```python
from build123d import *

# Parameters (mm, degrees)
F1_DEPTH = 60


# Not quite as in the source:
# - a feature names something its author has since deleted; it is built from what else it names


with BuildPart() as f1:
    # F0 (on Right) → F1 (new body)
    with BuildSketch(Plane.YZ):
        Polygon((-9.6511039816, 84.8569979519), (11.5631884334, -16.6570162717), (-54.0677122772, -34.3161821365), (58.7390847504, -34.3161821365), (57.1931600571, -30.1430020481), (52.030442059, -16.6570162717), (41.619012037, -7.4873352069), (45.6172674894, -16.6570162717), (45.6120451947, -16.6570162717), (34.6120451947, -16.6570162717), align=None)
        Polygon((-33.4832413232, -32.6066525748), (14.5474322128, -19.683142134), (1.6078982385, -32.6066525748), align=None, mode=Mode.SUBTRACT)
        Polygon((6.7093357808, -32.6066525748), (27.5331988357, -11.8085765279), (36.6017826139, -32.6066525748), align=None, mode=Mode.SUBTRACT)
        Polygon((34.5994135062, -18.9948312665), (45.6120451947, -18.9948312665), (49.0652749053, -18.9948312665), (54.2761653822, -32.6066525748), (40.534575087, -32.6066525748), (38.136206347, -27.1061845124), align=None, mode=Mode.SUBTRACT)
        Polygon((16.4317106992, -17.8011970237), (3.8088566841, 42.6013163841), (25.9855565835, -8.2591820422), align=None, mode=Mode.SUBTRACT)
    extrude(amount=F1_DEPTH)


solid = f1.part
```
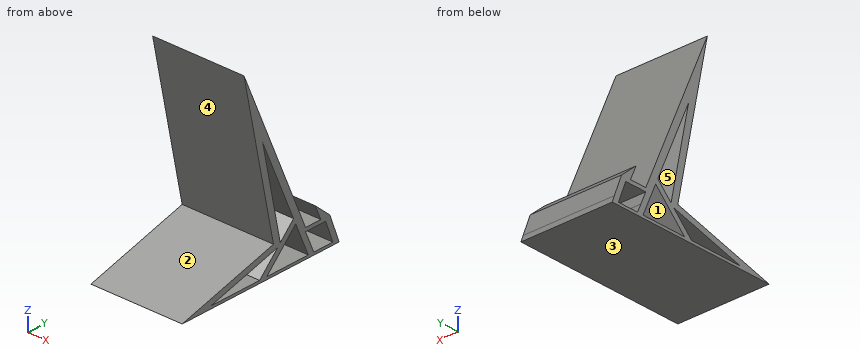
Geometry: final body of the model. Coordinates: model frame, mm. Face numbers are marked on the shaded views. A direction names the side the tool comes from. Round coordinates to 2 decimals unless told otherwise and drop trailing zeros. Order: outer loops, then holes, each group sorted by start corner. A loop starts at its lowest first (then second) coordinate and runs counter-clockwise, first axis right, second up. Notation, with made-up numbers: (-7, -13) -> (27, -13) arc R3 cw to (27, -9) -> close; hole circle Ø3 at (-18.75, 29.5). An arc over 180 degrees is marked (long way). Use one line per item in the form item = value. Start each with the question number.
1. Pin query (flat end, axial travel): pin 1 Ø4 at (x, y) = (47, -12) entering from +Z; pin 2 Ø6 at (x, z) = (8, 26) entering from -Y; pin 3 Ø4 at (x, y) = (44.5, 16.5) entering from +Z. Return the tip coordinate at first contact, or that it passes through.
2. Cut plane C-C (y = -6.5). Return the cut outline in (x, z), then the cut area to 3 significant figures.
3. Cut plane B-B (y = 13). Return the cut outline in (x, z), then the cut area to 3 significant figures.
4. Line query: probe 1 along Y at (x, z) = (45, -13); probe 2 along Z at (x, y) = (45, 25.5); probe 3 along Z at (x, y) = (20.5, -17). Output: solid intervals per line, ascending.
5. Draft query along Y for the marked faces 3, 4 and 5. Return one class per face: pulls with the +Y half, pulls with the -Y half, needs draft (parallel to the pull), parting line crosses it, or undercut.
6. Cut plane A-A (x = 45). Return the cut outline in (y, z).
7. Reachability of the marked faces 1 and 2 from +Z, -Z, +X, -X, +Y, -Y: full face, straight path, thin tool, end or side. Return the list, or none.
8. Cut plane D-D (z = 15.5). Return the cut outline in (x, y), then the cut area to 3 significant figures.
Solution:
q1.pin_1 = -22.46
q1.pin_2 = 2.02
q1.pin_3 = 29.47
q2.outline = (0, -34.32) -> (60, -34.32) -> (60, -32.61) -> (0, -32.61) -> close; (0, -25.35) -> (60, -25.35) -> (60, -21.52) -> (0, -21.52) -> close; (0, 69.78) -> (60, 69.78) -> (60, 77.63) -> (0, 77.63) -> close
q2.area = 803 mm^2
q3.outline = (0, -34.32) -> (60, -34.32) -> (60, -32.61) -> (0, -32.61) -> close; (0, -26.32) -> (60, -26.32) -> (60, -21.23) -> (0, -21.23) -> close; (0, -20.1) -> (60, -20.1) -> (60, -1.38) -> (0, -1.38) -> close; (0, 21.52) -> (60, 21.52) -> (60, 32.91) -> (0, 32.91) -> close
q3.area = 2,210 mm^2
q4.probe_1 = 10.8 to 15.43, 21.24 to 26.34, 28.05 to 33.02, 44.02 to 47.88
q4.probe_2 = -34.32 to -32.61, -13.84 to -8.74, -7.15 to 4.24
q4.probe_3 = -34.32 to -32.61, -28.17 to -24.34
q5.face_3 = needs draft
q5.face_4 = pulls with the -Y half
q5.face_5 = undercut
q6.outline = (-54.07, -34.32) -> (58.74, -34.32) -> (57.19, -30.14) -> (52.03, -16.66) -> (41.62, -7.49) -> (45.62, -16.66) -> (34.61, -16.66) -> (-9.65, 84.86) -> (11.56, -16.66) -> close; hole (-33.48, -32.61) -> (1.61, -32.61) -> (14.55, -19.68) -> close; hole (3.81, 42.6) -> (16.43, -17.8) -> (25.99, -8.26) -> close; hole (6.71, -32.61) -> (36.6, -32.61) -> (27.53, -11.81) -> close; hole (34.6, -18.99) -> (40.53, -32.61) -> (54.28, -32.61) -> (49.07, -18.99) -> close
q7.face_1 = +X, -X
q7.face_2 = +X, -X, -Y
q8.outline = (0, 4.84) -> (60, 4.84) -> (60, 9.47) -> (0, 9.47) -> close; (0, 15.63) -> (60, 15.63) -> (60, 20.59) -> (0, 20.59) -> close
q8.area = 576 mm^2
